from build123d import *

# Parameters (mm, degrees)
SKETCH_1_R      = 2.05
SKETCH_1_R_2    = 5.05
SKETCH_1_W      = 8.1
SKETCH_1_H      = 2.1
EXTRUDE_1_DEPTH = 2


with BuildPart() as part:
    # 草图1 → 凸台-拉伸1 (new body)
    with BuildSketch(Plane.XY):
        with BuildLine():
            ThreePointArc((-10.95, -11.95191036), (0, -4.124206955), (10.95, -11.95191036))
            ThreePointArc((10.95, -11.95191036), (0, 65.5), (-10.95, -11.95191036))
        make_face()
        Circle(SKETCH_1_R, mode=Mode.SUBTRACT)
        with Locations((0, 8)):
            Circle(SKETCH_1_R, mode=Mode.SUBTRACT)
        with Locations((0, 26)):
            Circle(SKETCH_1_R_2, mode=Mode.SUBTRACT)
        with Locations((-15, 8)):
            Rectangle(SKETCH_1_W, SKETCH_1_H, mode=Mode.SUBTRACT)
        with Locations((-15, 0)):
            Rectangle(SKETCH_1_W, SKETCH_1_H, mode=Mode.SUBTRACT)
        with Locations((15, 8)):
            Rectangle(SKETCH_1_W, SKETCH_1_H, mode=Mode.SUBTRACT)
        with Locations((15, 0)):
            Rectangle(SKETCH_1_W, SKETCH_1_H, mode=Mode.SUBTRACT)
    extrude(amount=EXTRUDE_1_DEPTH)


solid = part.part
The model under review builds one solid part; all positions refer to its coordinate system, in mm. A direction names the side the tool comes from. Coordinates: 2 decimals unless noted, no trailing zeros. Order: outer loops, then holes, each group sorted by start corner. A loop starts at its lowest first (then second) coordinate and runs counter-clockwise, first axis right, second up. Notation, with made-up numbers: (16.25, -40) -> (29.25, -40) arc R33 ccw to (29.25, -2) -> close; hole circle Ø1 at (-7, 17.5). An arc over 180 degrees is marked (long way). Answer in a Markdown table with one row per item.
(1) Consider section B-B (y = 26). Write out the cut boundary in (x, z).
Answers:
| item | result |
|---|---|
| outline | (-39.5, 0) -> (-5.05, 0) -> (-5.05, 2) -> (-39.5, 2) -> close; (5.05, 0) -> (39.5, 0) -> (39.5, 2) -> (5.05, 2) -> close |
(2) Consider section D-D (y = 0). Write out the cut boundary in (x, z), plus the area to 3 significant figures.
Answers:
| item | result |
|---|---|
| outline | (-29.74, 0) -> (-19.05, 0) -> (-19.05, 2) -> (-29.74, 2) -> close; (-10.95, 0) -> (-2.05, 0) -> (-2.05, 2) -> (-10.95, 2) -> close; (2.05, 0) -> (10.95, 0) -> (10.95, 2) -> (2.05, 2) -> close; (19.05, 0) -> (29.74, 0) -> (29.74, 2) -> (19.05, 2) -> close |
| area | 78.3 mm² |
(3) Machinability: for faces 1 (the flat face through (10.95, 0, 1)), 2 (the flat face through (-1, 19, 2)), which of the approach directions +Z, -Z, +X, -X, +Y, -Y give a long, thin tool a straight path to every point of the face, cutting with its end or side? Answer none if there is none.
Answers:
| item | result |
|---|---|
| face 1 | +Z, -Z |
| face 2 | +Z, +X, -X, +Y, -Y |
(4) Consider section C-C (z = 1.5). Write out the cut boundary in (x, y).
Answers:
| item | result |
|---|---|
| outline | (-10.95, -11.95) arc R11.57 cw to (10.95, -11.95) arc R39.5 ccw (long way) to start; hole (-19.05, -1.05) -> (-10.95, -1.05) -> (-10.95, 1.05) -> (-19.05, 1.05) -> close; hole (-19.05, 6.95) -> (-10.95, 6.95) -> (-10.95, 9.05) -> (-19.05, 9.05) -> close; hole circle Ø10.1 at (0, 26); hole circle Ø4.1 at (0, 0); hole circle Ø4.1 at (0, 8); hole (10.95, -1.05) -> (19.05, -1.05) -> (19.05, 1.05) -> (10.95, 1.05) -> close; hole (10.95, 6.95) -> (19.05, 6.95) -> (19.05, 9.05) -> (10.95, 9.05) -> close |
(5) Wall thickness on line 1 along Y through (x, z) = (0, 1.2); line 2 along Y through (x, z) = (19, 1.55); line 3 along X through (y, z) = (9, 0.9): over which ranges is each line inside the solid? List them lowest first.
Answers:
| item | result |
|---|---|
| line 1 | -4.12 to -2.05, 2.05 to 5.95, 10.05 to 20.95, 31.05 to 65.5 |
| line 2 | -8.63 to -1.05, 1.05 to 6.95, 9.05 to 60.63 |
| line 3 | -35.65 to -19.05, -10.95 to -1.79, 1.79 to 10.95, 19.05 to 35.65 |
(6) Insertion check: pin 1 (3.5 mm diameter, centred on x = 0, y = 8, fed in from +Z); pin 2 (0.6 mm diameter, centred on x = -16.5, z = 1, fed in from -Y); pin 3 (1 mm diameter, centred on y = 8.5, z = 1, fed in from +X); pin 4 (0.6 mm diameter, centred on x = -13, z = 1.5, fed in from -Y). Each pin has a flat end and moves straight along its axis. Give the tip position at first contact, or say it passes through.
Answers:
| item | result |
|---|---|
| pin 1 | through |
| pin 2 | y = -10.03 |
| pin 3 | x = 35.65 |
| pin 4 | y = -11.4 |
(7) Consider section A-A (x = 0). Write out the cut boundary in (y, z).
Answers:
| item | result |
|---|---|
| outline | (-4.12, 0) -> (-2.05, 0) -> (-2.05, 2) -> (-4.12, 2) -> close; (2.05, 0) -> (5.95, 0) -> (5.95, 2) -> (2.05, 2) -> close; (10.05, 0) -> (20.95, 0) -> (20.95, 2) -> (10.05, 2) -> close; (31.05, 0) -> (65.5, 0) -> (65.5, 2) -> (31.05, 2) -> close |
